Design review of the part built by this model. Coordinates are the model's own, in mm. Face numbers are marked on the shaded views. A direction names the side the tool comes from. Give positions to 0.01 mm unless a question says otherwise; leave off trailing zeros. Loops run counter-clockwise (first coordinate to the right, second up) from the corner with the lowest first, then second, coordinate; pieces in that order, holes last. Notation, with made-up numbers: M 89.5,21 L 115.5,21 A23 cw 115.5,49 Z; hole C -33.75,4 d9. An arc over 180 degrees is marked long. Use CSV: the item, a comma, the result in double quotes.
from build123d import *

# Parameters (mm, degrees)
CUT_EXTRUDE_5_DEPTH      = 34.271609519
CUT_EXTRUDE_5_DEPTH_BACK = 34.271609519
SKETCH_8_R               = 4
EXTRUDE_START            = -75
SKETCH_10_R              = 4
EXTRUDE_1_DEPTH          = 150
SKETCH_12_R              = 2.75
CUT_EXTRUDE_6_DEPTH      = 6
PATTERN_CIRCULAR_1_COUNT = 6


with BuildPart() as part:
    # 草图3 → 旋转1 (revolve)
    with BuildSketch(Plane(origin=(0, 0, 0), x_dir=(0, 0, -1), z_dir=(1, 0, 0)), mode=Mode.PRIVATE) as revolve_1_sk:
        Polygon((-3, 0), (-3, 21), (3, 21), (3, 11.75), (15, 11.75), (15, 0), align=None)
    revolve(revolve_1_sk.sketch.rotate(Axis((0, 0, 3), (0, 0, -1)), 90), axis=Axis((0, 0, 3), (0, 0, -1)))

    # 草图8 → 切除-拉伸5 (cut, two sides: drawn at the far end of the back side and taken through both)
    with BuildSketch(Plane.XY.offset(-CUT_EXTRUDE_5_DEPTH_BACK)):
        Circle(SKETCH_8_R)
    extrude(amount=CUT_EXTRUDE_5_DEPTH + CUT_EXTRUDE_5_DEPTH_BACK, mode=Mode.SUBTRACT)

    # 草图12 → 切除-拉伸6 (cut)
    with BuildSketch(Plane.XY.offset(3)):
        with Locations((16, 0)):
            Circle(SKETCH_12_R)
    cut_extrude_6 = extrude(amount=-CUT_EXTRUDE_6_DEPTH, mode=Mode.SUBTRACT)

    # 阵列(圆周)1: 切除-拉伸6 ×6 about axis
    pattern_circular_1_axis = Axis((0, 0, 0), (0, 0, 1))
    for i in range(1, PATTERN_CIRCULAR_1_COUNT):
        add(cut_extrude_6.rotate(pattern_circular_1_axis, i * 360 / PATTERN_CIRCULAR_1_COUNT), mode=Mode.SUBTRACT)


with BuildPart() as body_2:
    # 草图10 → 凸台-拉伸1 (new body)
    with BuildSketch(Plane.XY.offset(EXTRUDE_START)):
        Circle(SKETCH_10_R)
    extrude(amount=EXTRUDE_1_DEPTH)


solid = part.part
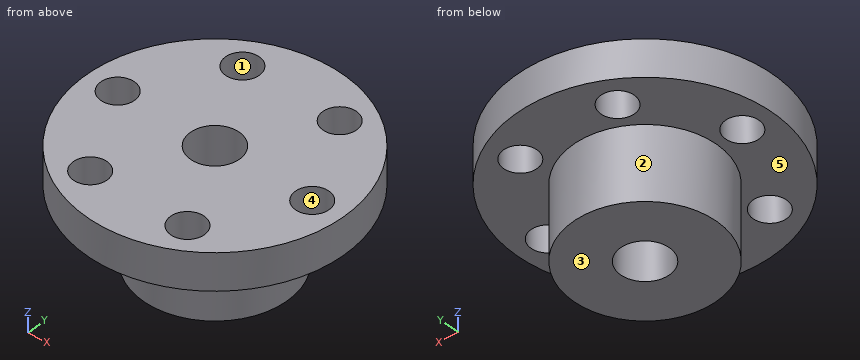
(1) The part is to be moulded in two halves that separate along Y. For the marked faces 1, 2 and 3, say which applies: released by +Y, released by -Y, zero draft, split by the parting line, or undercut.
A:
face 1,"undercut"
face 2,"split by the parting line"
face 3,"zero draft"
(2) Machinability: for the marked faces 4 and 5, which of the approach directions +Z, -Z, +X, -X, +Y, -Y give a long, thin tool a straight path to every point of the face, cutting with its end or side? Answer none if there is none.
A:
face 4,"+Z, -Z"
face 5,"-Z"
(3) We need section B-B on y = 0. State the section outline as (x, z) points, then the cut area to 3 significant figures.
A:
outline,"M -21,-3 L -18.75,-3 L -18.75,3 L -21,3 Z; M -13.25,-3 L -11.75,-3 L -11.75,-15 L -4,-15 L -4,3 L -13.25,3 Z; M 4,-15 L 11.75,-15 L 11.75,-3 L 13.25,-3 L 13.25,3 L 4,3 Z; M 18.75,-3 L 21,-3 L 21,3 L 18.75,3 Z"
area,"324 mm²"
(4) We need section D-D on z = 1. State the section outline as (x, y) points (3 decimals).
A:
outline,"C 0,0 d42; hole C -16,0 d5.5; hole C -8,-13.856 d5.5; hole C -8,13.856 d5.5; hole C 0,0 d8; hole C 8,-13.856 d5.5; hole C 8,13.856 d5.5; hole C 16,0 d5.5"
(5) We need section C-C on x = -8. State the section outline as (y, z) points, then the cut area to 3 significant figures.
A:
outline,"M -19.42,-3 L -16.61,-3 L -16.61,3 L -19.42,3 Z; M -11.11,-3 L -8.61,-3 L -8.61,-15 L 8.61,-15 L 8.61,-3 L 11.11,-3 L 11.11,3 L -11.11,3 Z; M 16.61,-3 L 19.42,-3 L 19.42,3 L 16.61,3 Z"
area,"374 mm²"
(6) Wall thickness on line 1 along Y through (x, z) = (-8, -1.25); line 2 along Y through (x, z) = (0, -8.25); line 3 along Y through (x, z) = (-6.5, -0.25): over which ranges is each line inside the solid? List them lowest first. Write a range as [from, to].
A:
line 1,"[-19.42, -16.61], [-11.11, 11.11], [16.61, 19.42]"
line 2,"[-11.75, -4], [4, 11.75]"
line 3,"[-19.97, -16.16], [-11.55, 11.55], [16.16, 19.97]"
(7) We need section A-A on x = 0. State the section outline as (y, z) points.
A:
outline,"M -21,-3 L -11.75,-3 L -11.75,-15 L -4,-15 L -4,3 L -21,3 Z; M 4,-15 L 11.75,-15 L 11.75,-3 L 21,-3 L 21,3 L 4,3 Z"
(8) Clearance check with flat-ended pins moving along their axes: P1, Ø1.5, axis at x = -6.5, z = -12.5, coming from the +Y side; P2, Ø10, axis at x = -7.5, z = -10.5, coming from the +Y side; P3, Ø7, axis at x = -8, y = -13.86, coming from the -Z side. State where each tip first meets the part, or that it passes through.
A:
P1,"y = 10.25"
P2,"y = 11.48"
P3,"z = -3"
